For this review, take the finished solid that the model builds, in its own axes (mm). Face numbers are marked on the shaded views. A direction names the side the tool comes from. Give positions to 0.01 mm unless a question says otherwise; leave off trailing zeros. Write each loop counter-clockwise with the first axis right and the second up, starting at its lowest first coordinate (ties: lowest second). Pieces come first, ordered by that corner, then holes.
1) Draft analysis for pull direction Y (two halves, no side actions). For the marked faces 4, 5 and 6, state which applies: pulls with the +Y half, pulls with the -Y half, needs draft (parallel to the pull), parting line crosses it, or undercut.
2) Wall thickness on line 1 along X through (y, z) = (32, -85); line 2 along Y through (x, z) = (188.5, 211.5); line 3 along Z through (x, y) = (-18.5, 160): over which ranges is each line inside the solid? List them lowest first.
3) We need section C-C on x = -153. Give the boundary of the cut face in (y, z).
4) We need section A-A on y = 0. Give the boundary of the cut face in (x, z), and give its area (3 significant figures).
5) We need section D-D on y = 144.5. Give the boundary of the cut face in (x, z).
6) Machinability: for the marked faces 1, 2 and 3, which of the approach directions +Z, -Z, +X, -X, +Y, -Y give a long, thin tool a straight path to every point of the face, cutting with its end or side? Answer none if there is none.
7) We need section B-B on z = 56. Give the boundary of the cut face in (x, y), and give its area (3 significant figures).
8) For P1, Ø0.9, axis at y = 198.5, z = -14.5, coming from the +X side; P2, Ø3.5, axis at y = -198.5, z = -8, coming from the +X side; P3, Ø1, axis at x = 125, y = -152, coming from the -Z side, all flat-tipped, find the tip position at first contact; note any pin that passes through.
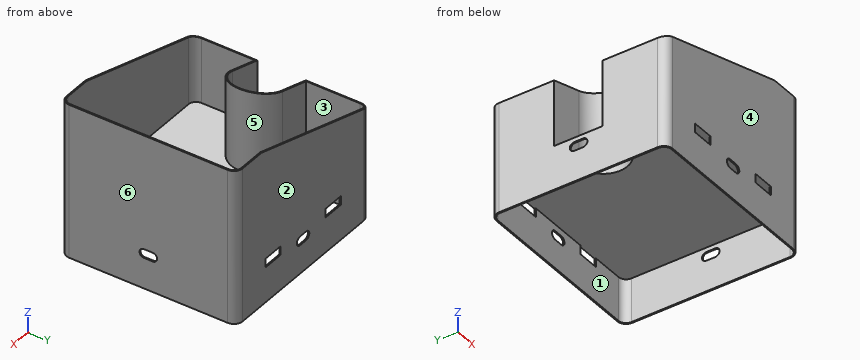
from build123d import *

# Parameters (mm, degrees)
EXTRUDE_1_DEPTH     = 250
SHELL_1_T           = -3
CUT_EXTRUDE_1_DEPTH = 547
EXTRUDE_START       = 100
EXTRUDE_3_DEPTH     = 100
SKETCH_6_W          = 50
SKETCH_6_H          = 20
CUT_EXTRUDE_3_DEPTH = 472
SKETCH_7_W          = 20
SKETCH_7_H          = 40
CUT_EXTRUDE_4_DEPTH = 472
FILLET_1_R          = 10
FILLET_2_R          = 10
CUT_EXTRUDE_5_DEPTH = 472


with BuildPart() as part:
    # 草图1 → 凸台-拉伸1 (new body)
    with BuildSketch(Plane.XY):
        with BuildLine():
            Line((-135, 55), (-215, 55))
            Line((-215, 55), (-215, 180))
            ThreePointArc((-215, 180), (-209.142135624, 194.142135624), (-195, 200))
            Line((-195, 200), (195, 200))
            ThreePointArc((195, 200), (209.142135624, 194.142135624), (215, 180))
            Line((215, 180), (215, -180))
            ThreePointArc((215, -180), (209.142135624, -194.142135624), (195, -200))
            Line((195, -200), (-195, -200))
            ThreePointArc((-195, -200), (-209.142135624, -194.142135624), (-215, -180))
            Line((-215, -180), (-215, -55))
            Line((-215, -55), (-135, -55))
            ThreePointArc((-135, -55), (-80, 0), (-135, 55))
        make_face()
    extrude(amount=EXTRUDE_1_DEPTH)

    # 抽壳1
    shell_1_openings = [part.faces().sort_by_distance(p)[0] for p in [
        (13.096091643, 0, 250),
    ]]
    offset(amount=SHELL_1_T, openings=shell_1_openings, kind=Kind.INTERSECTION)

    # 草图3 → 切除-拉伸1 (cut)
    with BuildSketch(Plane(origin=(0, 200, 0), x_dir=(1, 0, 0), z_dir=(0, 1, 0))):
        Polygon((134.47381547, -250), (-215.52618453, -150), (-215.52618453, -250), align=None)
    extrude(amount=-CUT_EXTRUDE_1_DEPTH, mode=Mode.SUBTRACT)

    # 草图4 → 凸台-拉伸3 (add)
    with BuildSketch(Plane(origin=(0, 0, 0), x_dir=(-1, 0, 0), z_dir=(0, 0, -1)).offset(EXTRUDE_START)):
        with BuildLine():
            Line((195, -200), (-195, -200))
            ThreePointArc((-195, -200), (-209.142135624, -194.142135624), (-215, -180))
            Line((-215, -180), (-215, 180))
            ThreePointArc((-215, 180), (-209.142135624, 194.142135624), (-195, 200))
            Line((-195, 200), (195, 200))
            ThreePointArc((195, 200), (209.142135624, 194.142135624), (215, 180))
            Line((215, 180), (215, -180))
            ThreePointArc((215, -180), (209.142135624, -194.142135624), (195, -200))
        make_face()
        with BuildLine():
            Line((195, -197), (-195, -197))
            ThreePointArc((-195, -197), (-207.02081528, -192.02081528), (-212, -180))
            Line((-212, -180), (-212, 180))
            ThreePointArc((-212, 180), (-207.02081528, 192.02081528), (-195, 197))
            Line((-195, 197), (195, 197))
            ThreePointArc((195, 197), (207.02081528, 192.02081528), (212, 180))
            Line((212, 180), (212, -180))
            ThreePointArc((212, -180), (207.02081528, -192.02081528), (195, -197))
        make_face(mode=Mode.SUBTRACT)
    extrude(amount=-EXTRUDE_3_DEPTH)

    # 草图6 → 切除-拉伸3 (cut)
    with BuildSketch(Plane(origin=(0, 200, 0), x_dir=(1, 0, 0), z_dir=(0, 1, 0))):
        with Locations((-97.377223929, 10)):
            Rectangle(SKETCH_6_W, SKETCH_6_H)
        with Locations((97.246218359, 10)):
            Rectangle(SKETCH_6_W, SKETCH_6_H)
    extrude(amount=-CUT_EXTRUDE_3_DEPTH, mode=Mode.SUBTRACT)

    # 草图7 → 切除-拉伸4 (cut)
    with BuildSketch(Plane.ZY.offset(215)):
        with Locations((-20, -0.350965312)):
            Rectangle(SKETCH_7_W, SKETCH_7_H)
    extrude(amount=-CUT_EXTRUDE_4_DEPTH, mode=Mode.SUBTRACT)

    # 圆角1
    fillet_1_edges = [part.edges().sort_by_distance(p)[0] for p in [
        (-213.5, -20.350965312, -30),
        (-213.5, -20.350965312, -10),
        (-213.5, 19.649034688, -10),
        (-213.5, 19.649034688, -30),
    ]]
    fillet(fillet_1_edges, radius=FILLET_1_R - 0.0001)  # a hair under: the kernel refuses the full size

    # 圆角2
    fillet_2_edges = [part.edges().sort_by_distance(p)[0] for p in [
        (213.5, -20.350965312, -30),
        (213.5, 19.649034688, -30),
        (213.5, 19.649034688, -10),
        (213.5, -20.350965312, -10),
    ]]
    fillet(fillet_2_edges, radius=FILLET_2_R - 0.0001)  # a hair under: the kernel refuses the full size

    # 草图8 → 切除-拉伸5 (cut)
    with BuildSketch(Plane(origin=(0, 200, 0), x_dir=(1, 0, 0), z_dir=(0, 1, 0))):
        with BuildLine():
            Line((10.1, 15), (-10.1, 15))
            ThreePointArc((-10.1, 15), (-17.100357134, 17.899642866), (-20, 24.9))
            Line((-20, 24.9), (-20, 25.1))
            ThreePointArc((-20, 25.1), (-17.100357134, 32.100357134), (-10.1, 35))
            Line((-10.1, 35), (10.1, 35))
            ThreePointArc((10.1, 35), (17.100357134, 32.100357134), (20, 25.1))
            Line((20, 25.1), (20, 24.9))
            ThreePointArc((20, 24.9), (17.100357134, 17.899642866), (10.1, 15))
        make_face()
    extrude(amount=-CUT_EXTRUDE_5_DEPTH, mode=Mode.SUBTRACT)


solid = part.part
Results list:
1. face 4: pulls with the -Y half
1. face 5: undercut
1. face 6: needs draft
2. line 1: x = -215 to -212, 212 to 215
2. line 2: y = -200 to -197, 197 to 200
2. line 3: z = 0 to 3
3. outline: (-200, -100) - (-197, -100) - (-197, 0) - (-55, 0) - (-55, 167.86) - (-58, 167.86) - (-58, 3) - (-197, 3) - (-197, 167.86) - (-200, 167.86) - close; (55, 0) - (197, 0) - (197, -100) - (200, -100) - (200, 167.86) - (197, 167.86) - (197, 3) - (58, 3) - (58, 167.86) - (55, 167.86) - close
4. outline: (-215, -100) - (-212, -100) - (-212, -30) - (-215, -30) - close; (-215, -10) - (-212, -10) - (-212, 0) - (-215, 0) - close; (-80, 0) - (212, 0) - (212, -10) - (215, -10) - (215, 250) - (212, 250) - (212, 3) - (-77, 3) - (-77, 189.58) - (-80, 188.72) - close; (212, -100) - (215, -100) - (215, -30) - (212, -30) - close
4. area: 2,660 mm2
5. outline: (-215, -100) - (-212, -100) - (-212, 0) - (212, 0) - (212, -100) - (215, -100) - (215, 250) - (212, 250) - (212, 3) - (-212, 3) - (-212, 151.01) - (-215, 150.15) - close
6. face 1: -Z
6. face 2: +Z, -Z, +X, -X, +Y
6. face 3: +Z
7. outline: (-215, -180) arc R20 ccw to (-195, -200) - (195, -200) arc R20 ccw to (215, -180) - (215, 180) arc R20 ccw to (195, 200) - (-195, 200) arc R20 ccw to (-215, 180) - (-215, 55) - (-135, 55) arc R55 cw to (-135, -55) - (-215, -55) - close; hole (-212, -180) arc R17 ccw to (-195, -197) - (195, -197) arc R17 ccw to (212, -180) - (212, 180) arc R17 ccw to (195, 197) - (-195, 197) arc R17 ccw to (-212, 180) - (-212, 58) - (-135, 58) arc R58 cw to (-135, -58) - (-212, -58) - close
7. area: 5,510 mm2
8. P1: stops at x = 203.61
8. P2: stops at x = 205.93
8. P3: stops at z = 0
